from build123d import *

# Parameters (mm, degrees)
SKETCH1_R           = 125
BOSS_EXTRUDE1_DEPTH = 250
SKETCH2_R           = 155
BOSS_EXTRUDE2_DEPTH = 20
SKETCH3_R           = 30
CUT_EXTRUDE1_DEPTH  = 364.524414586


with BuildPart() as part:
    # Sketch1 → Boss-Extrude1 (new body)
    with BuildSketch(Plane(origin=(0, 0, 0), x_dir=(0, 0, -1), z_dir=(1, 0, 0))):
        Circle(SKETCH1_R)
    extrude(amount=BOSS_EXTRUDE1_DEPTH)

    # Sketch2 → Boss-Extrude2 (add)
    with BuildSketch(Plane(origin=(0, 0, 0), x_dir=(0, 0, -1), z_dir=(1, 0, 0))):
        Circle(SKETCH2_R)
    boss_extrude2 = extrude(amount=-BOSS_EXTRUDE2_DEPTH)

    # Mirror1: Boss-Extrude2 across plane
    add(boss_extrude2.mirror(Plane(origin=(125, 0, 0), x_dir=(0, 0, 1), z_dir=(1, 0, 0))))

    # Sketch3 → Cut-Extrude1 (cut, through all)
    with BuildSketch(Plane.ZY.offset(20)):
        Circle(SKETCH3_R)
    extrude(amount=-CUT_EXTRUDE1_DEPTH, mode=Mode.SUBTRACT)


solid = part.part
Design review of the part built by this model. Coordinates are the model's own, in mm. A direction names the side the tool comes from. Coordinates: 2 decimals unless noted, no trailing zeros. Write each loop counter-clockwise with the first axis right and the second up, starting at its lowest first coordinate (ties: lowest second). Pieces come first, ordered by that corner, then holes. Notation, with made-up numbers: (2.25, 48) - (15.25, 48) arc R33 ccw to (15.25, 76) - close; hole circle Ø2 at (1.25, 36). An arc over 180 degrees is marked (long way). Use one line per item in the form item = value.
Q1. Consider section C-C (z = -36.5). Write out the cut boundary in (x, y).
Taken from the geometry:
outline = (-20, -150.64) - (0, -150.64) - (0, -119.55) - (250, -119.55) - (250, -150.64) - (270, -150.64) - (270, 150.64) - (250, 150.64) - (250, 119.55) - (0, 119.55) - (0, 150.64) - (-20, 150.64) - close
Q2. Consider section D-D (x = 33.5). Write out the cut boundary in (y, z).
Taken from the geometry:
outline = circle Ø250 at (0, 0); hole circle Ø60 at (0, 0)
Q3. Consider section A-A (y = 0). Write out the cut boundary in (x, z).
Taken from the geometry:
outline = (-20, -155) - (0, -155) - (0, -125) - (250, -125) - (250, -155) - (270, -155) - (270, -30) - (-20, -30) - close; (-20, 30) - (270, 30) - (270, 155) - (250, 155) - (250, 125) - (0, 125) - (0, 155) - (-20, 155) - close
Q4. The part is to be moulded in two halves that separate along X. For faces 3 (the flat face through (250, 70, 104)), 4 (the flat face through (270, -32, 2)), 5 (the cylindrical face through (-9.86, -151.314, 33.601)), 6 (the flat face through (-20, -32, 2)), say which applies: +X half, -X half, draft (parallel to the pull), parting line (faces both ways), or undercut.
Taken from the geometry:
face_3 = undercut
face_4 = +X half
face_5 = draft
face_6 = -X half
Q5. Machinability: for faces 1 (the flat face through (0, 70, 104)), 2 (the cylindrical face through (122.97, 1.32, -29.97)), which of the approach directions +Z, -Z, +X, -X, +Y, -Y give a long, thin tool a straight path to every point of the face, cutting with its end or side? Answer none if there is none.
Taken from the geometry:
face_1 = none
face_2 = +X, -X
Q6. Insertion check: pin 1 Ø6 at (x, y) = (199.5, 7.5) entering from -Z; pin 2 Ø2 at (x, y) = (228.5, -90) entering from -Z; pin 3 Ø1.5 at (x, y) = (62, -97) entering from +Z. Each pin has a flat end and moves straight along its axis. Give the tip position at first contact, or say it passes through.
Taken from the geometry:
pin_1 = -124.92
pin_2 = -87.77
pin_3 = 79.76
Q7. For probe 1 along X at (y, z) = (-94.5, -87); probe 2 along Z at (x, y) = (107, 20); probe 3 along Z at (x, y) = (140.5, 100), list the stretches that pass through material, from the lowest coordinate up.
Taken from the geometry:
probe_1 = -20 to 0, 250 to 270
probe_2 = -123.39 to -22.36, 22.36 to 123.39
probe_3 = -75 to 75
